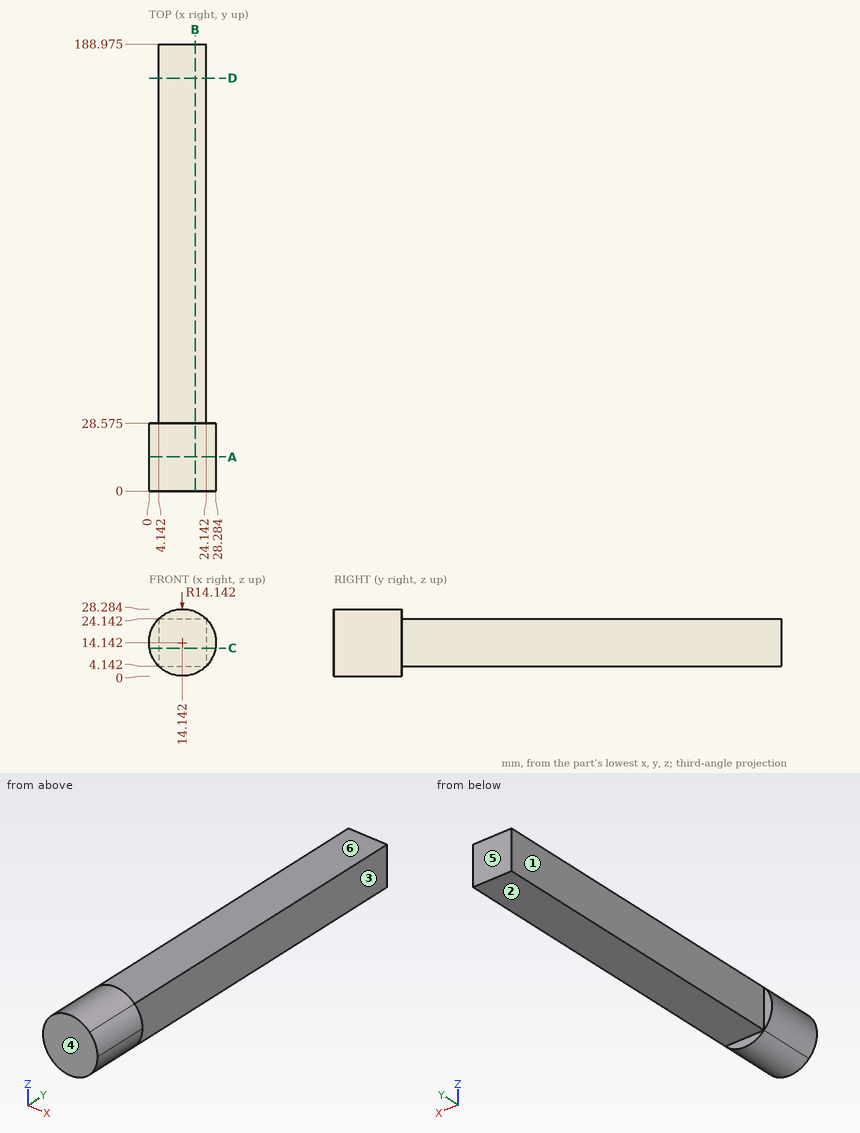
Can you work these out from the drawing? Everything is in mm from the part's minimum corner. A direction names the side the tool comes from. Round coordinates to 2 decimals unless told otherwise and drop trailing zeros. Loops run counter-clockwise (first coordinate to the right, second up) from the corner with the lowest first, then second, coordinate; pieces in that order, holes last.
1. If I drill on line 1 along Z through (x, y) = (21.75, 148.5); line 2 along X through (y, z) = (12, 13.75) (1 decimal), over which ranges is the centre line in solid material (lowest first)?
Answer list:
line 1: z = 4.14 to 24.14
line 2: x = 0 to 28.3
2. If we section it at D-D on y = 174.5: Write out the boundary of the cut face in (x, z).
Answer list:
outline: (4.14, 4.14) - (24.14, 4.14) - (24.14, 24.14) - (4.14, 24.14) - close
3. Which directions (+Z, -Z, +X, -X, +Y, -Y) give clear straight access to the entire face, cutting with the end or side of a thin tool? Please do the marked faces 1, 2 and 3.
Answer list:
face 1: +Z, -Z, -X, +Y
face 2: -Z, +X, -X, +Y
face 3: +Z, -Z, +X, +Y
4. For P1, Ø4, axis at y = 104.5, z = 5.5, coming from the -X side; P2, Ø1, axis at y = 140, z = 9, coming from the +X side; P3, Ø10, axis at x = 18, y = 109.5, coming from the -Z side, each with a flat end and sliding along its axis, tell me the tip position at first contact or that it passes through.
Answer list:
P1: stops at x = 4.14
P2: stops at x = 24.14
P3: stops at z = 4.14
5. If we section it at C-C on z = 11.75: Write out the boundary of the cut face in (x, y) (1 decimal).
Answer list:
outline: (0.2, 0) - (28.1, 0) - (28.1, 28.6) - (24.1, 28.6) - (24.1, 189) - (4.1, 189) - (4.1, 28.6) - (0.2, 28.6) - close
6. If we section it at B-B on x = 19.5: Write out the boundary of the cut face in (y, z) (1 decimal).
Answer list:
outline: (0, 1.1) - (28.6, 1.1) - (28.6, 4.1) - (189, 4.1) - (189, 24.1) - (28.6, 24.1) - (28.6, 27.2) - (0, 27.2) - close
7. If we section it at A-A on y = 14.5: Write out the boundary of the cut face in (x, z).
Answer list:
outline: circle Ø28.28 at (14.14, 14.14)
8. We'd pull the mould along Y, two halves only. Please class the marked faces 4, 5 and 6: +Y half, -Y half, draft (parallel to the pull), parting line (faces both ways), or undercut.
Answer list:
face 4: -Y half
face 5: +Y half
face 6: draft
